For this review, use the dimensioned drawing (mm, ordinates from the lowest corner) and the shaded views. Round coordinates to 2 decimals unless told otherwise and drop trailing zeros. Loops run counter-clockwise (first coordinate to the right, second up) from the corner with the lowest first, then second, coordinate; pieces in that order, holes last. Notation, with made-up numbers: (37.5, -8.5) -> (64.5, -8.5) arc R15 cw to (64.5, 10.5) -> close; hole circle Ø5 at (72.25, 33). An arc over 180 degrees is marked (long way). Write each question's results on one line, items separated by ' | '. Start each with the question number.
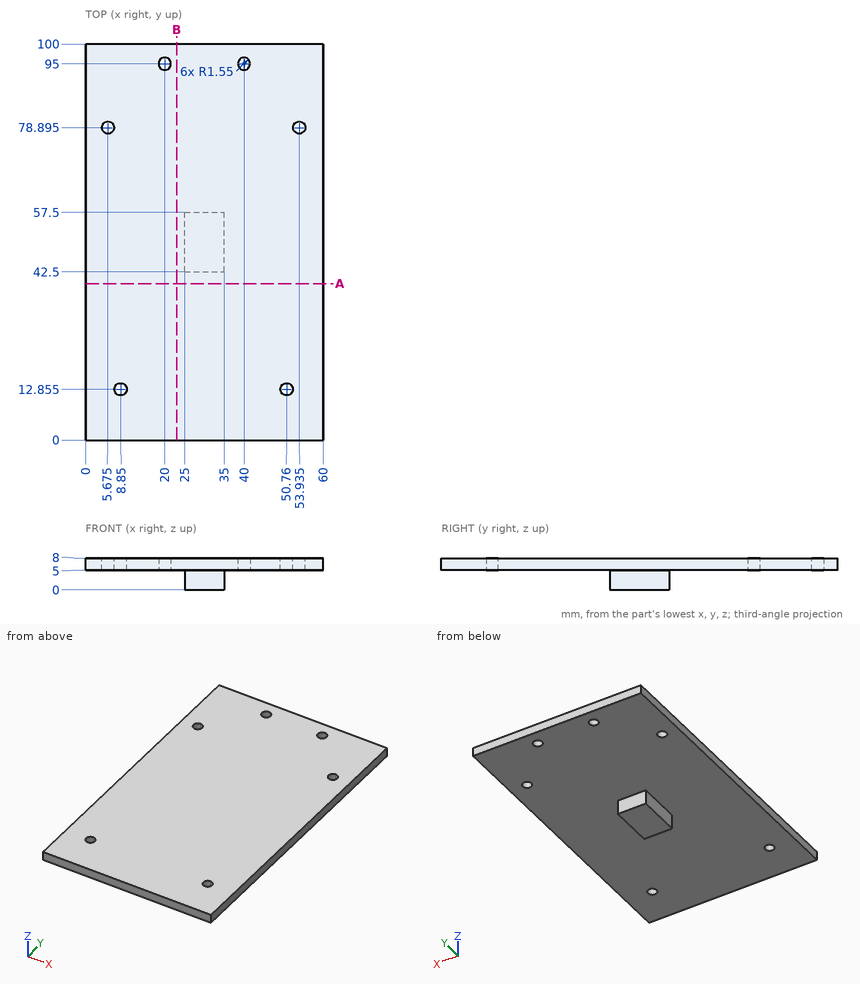
1) Take a section at A-A (y = 39.5). Write out the cut boundary in (x, z).
2) Insertion check: pin 1 (1.5 mm diameter, centred on y = 48.5, z = 3.5, fed in from +X); pin 2 (4 mm diameter, centred on y = 48, z = 2, fed in from -X); pin 3 (1.5 mm diameter, centred on x = 41, y = 28.5, fed in from -Z). Each pin has a flat end and moves straight along its axis. Give the tip position at first contact, or say it passes through.
3) To check wall thickness, follow line 1 (Z direction, x = 36, y = 56); line 2 (Y direction, x = 25.5, z = 3); line 3 (Y direction, x = 50, z = 6.25). State the ranges of each line that lie inside material, in increasing order. Write a range as from..to.
4) Take a section at B-B (x = 23). Write out the cut boundary in (y, z).
Geometry check:
1) outline: (0, 5) -> (60, 5) -> (60, 8) -> (0, 8) -> close
2) pin 1: stops at x = 35 | pin 2: stops at x = 25 | pin 3: stops at z = 5
3) line 1: z = 5..8 | line 2: y = 42.5..57.5 | line 3: y = 0..11.5, 14.21..100
4) outline: (0, 5) -> (100, 5) -> (100, 8) -> (0, 8) -> close
